CAD build for the part. Positions are in the model's coordinates, mm. Round coordinates to 2 decimals unless told otherwise and drop trailing zeros. Order: outer loops, then holes, each group sorted by start corner. A loop starts at its lowest first (then second) coordinate and runs counter-clockwise, first axis right, second up. Notation, with made-up numbers: (70.25, 65) - (88.25, 65) arc R14 ccw to (88.25, 84) - close; hole circle Ø10 at (1.25, -33.5). An arc over 180 degrees is marked (long way). Use one line per item in the form item = value. Start each with the question number.
Autodesk Inventor part; units mm, degrees
ref_plane "YZ Plane" through (0, 0, 0) normal (1, 0, 0) x (0, 1, 0)
ref_plane "XZ Plane" through (0, 0, 0) normal (0, 1, 0) x (-1, 0, 0)
ref_plane "XY Plane" through (0, 0, 0) normal (0, 0, 1) x (1, 0, 0)
sketch "Sketch1" plane through (0, 0, 0) normal (0, 0, 1) x (1, 0, 0)
  line L0 (0, 0) -> (25, 0)
  line L1 (25, 0) -> (25, 3)
  line L2 (0, 3) -> (25, 3)
  line L3 (0, 0) -> (0, 3)
  line L4 (0.2071, -72) -> (11, -72)
  line L5 (0.2071, -69) -> (11, -69)
  line L6 (25, -69) -> (50, -69)
  line L7 (25, 0) -> (50, 0)
  line L8 (-25, 0) -> (0, 0)
  line L9 (-22, 0) -> (-22, -10.8146)
  line L10 (-25, -22) -> (-25, -47)
  line L11 (-25, -47) -> (-22, -47)
  line L12 (-22, -10.8146) -> (-22, -58.1854)
  line L13 (-25, -22) -> (-22, -22)
  line L14 (-22, -58.1854) -> (-22, -69)
  line L15 (-25, -69) -> (0, -69)
  line L16 (50, 0) -> (50, -22)
  line L17 (50, -22) -> (47, -22)
  line L18 (47, -22) -> (47, -47)
  line L19 (47, -47) -> (50, -47)
  line L20 (50, -47) -> (50, -69)
  line L21 (50, 0) -> (25, 0)
  line L22 (25, 3) -> (25, 0)
  line L23 (25, 3) -> (0, 3)
  line L24 (0, 3) -> (0, 0)
  line L25 (-22, -10.8146) -> (-22, 0)
  line L26 (-22, 0) -> (0, 0)
  line L27 (-22, -22) -> (-25, -22)
  line L28 (-25, -22) -> (-25, -47)
  line L29 (-22, -47) -> (-25, -47)
  line L30 (-22, -58.1854) -> (-22, -69)
  line L31 (-22, -69) -> (0, -69)
  line L32 (0, -72) -> (0, -69)
  line L33 (0, -72) -> (25, -72)
  line L34 (25, -72) -> (25, -69)
  line L35 (25, -69) -> (50, -69)
  line L36 (11, -72) -> (11, -69)
  line L37 (0.2071, -69) -> (0.2071, -72)
  dimension "d0" = 3
extrude "Extrusion1" add sketch "Sketch1" along normal blind 3
sketch "Sketch2" plane through (0, 0, 3) normal (0, 0, 1) x (1, 0, 0)
  line L0 (-25, -22) -> (-25, -47)
  line L1 (-25, -34.5) -> (7, -34.5)
  line L2 (-25, -34.5) -> (-14, -34.5)
  circle A0 centre (-14, -34.5) radius 21
  circle A1 centre (-14, -34.5) radius 25
  point P0 (0, 0)
  dimension "d3" = 32
  dimension "d4" = 11
  dimension "d5" = 4
extrude "Extrusion2" cut sketch "Sketch2" against normal blind 20 contours A0 | A1
sketch "Sketch3" plane through (0, 0, 3) normal (0, 0, 1) x (1, 0, 0)
  line L0 (-1.2929, -65) -> (30.2929, -65)
  line L1 (-4.5, -67) -> (-4.5, -65)
  line L2 (33.5, -67) -> (33.5, -65)
  line L3 (30.6464, -65) -> (33.5, -65)
  line L4 (30.6464, -65) -> (30.2929, -65)
  line L5 (30.2929, -67) -> (30.6464, -67)
  line L6 (33.5, -67) -> (30.6464, -67)
  line L7 (30.2929, -67) -> (-1.2929, -67)
  arc A0 (-22, -58.1854) -> (-22, -10.8146) centre (-14, -34.5) ccw
  line L8 (-22, -58.1854) -> (-22, -69)
  line L9 (-22, -69) -> (0, -69)
  line L10 (0, -69) -> (0, -72)
  line L11 (50, -69) -> (50, -47)
  line L12 (50, -47) -> (47, -47)
  line L13 (47, -47) -> (47, -22)
  line L14 (47, -22) -> (50, -22)
  line L15 (50, -22) -> (50, 0)
  line L16 (50, 0) -> (25, 0)
  line L17 (25, 0) -> (25, 3)
  line L18 (25, 3) -> (0, 3)
  line L19 (0, 3) -> (0, 0)
  line L20 (0, 0) -> (-22, 0)
  line L21 (-22, 0) -> (-22, -10.8146)
  line L22 (-4.5, -65) -> (-1.6464, -65)
  line L23 (-1.2929, -65) -> (-1.6464, -65)
  line L24 (-1.6464, -67) -> (-4.5, -67)
  line L25 (-1.6464, -67) -> (-1.2929, -67)
  line L26 (0, -72) -> (25, -72)
  line L27 (25, -69) -> (50, -69)
  line L28 (25, -72) -> (25, -69)
extrude "Extrusion3" cut sketch "Sketch3" against normal blind 3 contours L0 L4 L3 L2 L6 L5 L7 L25 L24 L1 L22 L23
sketch "Sketch4" plane through (0, 0, 3) normal (0, 0, 1) x (1, 0, 0)
  line L0 (47, -47) -> (47, -22)
  line L1 (47, -34.5) -> (34.3, -34.5)
  line L2 (34.3, -34.5) -> (34.3, -36)
  line L3 (34.3, -36) -> (34.3, -33)
  line L4 (34.3, -33) -> (47, -33)
  line L5 (47, -33) -> (47, -36)
  line L6 (47, -36) -> (34.3, -36)
  line L7 (40.65, -36) -> (40.65, -38)
  line L8 (40.65, -38) -> (38.15, -38)
  line L9 (38.15, -38) -> (38.15, -31)
  line L10 (38.15, -31) -> (40.65, -31)
  line L11 (40.65, -31) -> (40.65, -36)
  line L12 (25, 3) -> (0, 3)
  line L13 (50, 0) -> (25, 0)
  line L14 (0, 0) -> (-22, 0)
  line L15 (25, -69) -> (50, -69)
  line L16 (0, -72) -> (25, -72)
  line L17 (-22, -69) -> (0, -69)
  line L18 (50, 0) -> (25, 0)
  line L19 (37.5, 0) -> (37.5, -12.7)
  line L20 (37.5, -12.7) -> (39, -12.7)
  line L21 (39, -12.7) -> (36, -12.7)
  line L22 (36, -12.7) -> (36, 0)
  line L23 (39, 0) -> (39, -12.7)
  line L24 (36, -6.35) -> (34, -6.35)
  line L25 (34, -6.35) -> (34, -8.85)
  line L26 (34, -8.85) -> (41, -8.85)
  line L27 (41, -8.85) -> (41, -6.35)
  line L28 (41, -6.35) -> (36, -6.35)
  line L29 (50, -69) -> (25, -69)
  line L30 (37.5, -69) -> (37.5, -56.3)
  line L31 (37.5, -56.3) -> (39, -56.3)
  line L32 (39, -56.3) -> (36, -56.3)
  line L33 (36, -56.3) -> (36, -69)
  line L34 (39, -69) -> (39, -56.3)
  line L35 (36, -62.65) -> (34, -62.65)
  line L36 (34, -62.65) -> (34, -60.15)
  line L37 (34, -60.15) -> (41, -60.15)
  line L38 (41, -60.15) -> (41, -62.65)
  line L39 (41, -62.65) -> (36, -62.65)
  line L40 (-4.5, -65) -> (33.5, -65)
  line L41 (33.5, -65) -> (33.5, -67)
  line L42 (33.5, -67) -> (-4.5, -67)
  line L43 (-4.5, -67) -> (-4.5, -65)
  arc A0 (-22, -58.1854) -> (-22, -10.8146) centre (-14, -34.5) ccw
  line L44 (-22, -58.1854) -> (-22, -69)
  line L45 (-22, -69) -> (0, -69)
  line L46 (0, -69) -> (0, -72)
  line L47 (0, -72) -> (25, -72)
  line L48 (25, -69) -> (50, -69)
  line L49 (50, -69) -> (50, -47)
  line L50 (50, -47) -> (47, -47)
  line L51 (47, -47) -> (47, -22)
  line L52 (47, -22) -> (50, -22)
  line L53 (50, -22) -> (50, 0)
  line L54 (50, 0) -> (25, 0)
  line L55 (25, 0) -> (25, 3)
  line L56 (25, 3) -> (0, 3)
  line L57 (0, 3) -> (0, 0)
  line L58 (0, 0) -> (-22, 0)
  line L59 (-22, 0) -> (-22, -10.8146)
  circle A1 centre (12.5, 1.5) radius 1.5
  line L60 (39, -56.3) -> (36, -56.3)
  line L61 (36, -56.3) -> (36, -69)
  line L62 (36, -69) -> (39, -69)
  line L63 (39, -69) -> (39, -56.3)
  circle A2 centre (12.5, -70.5) radius 1.5
  line L64 (25, -72) -> (25, -69)
  arc A3 (42.9741, -36.0257) -> (30.0259, -20.7829) centre (36.5, -28.4043) ccw
  line L65 (26.9692, -49.6214) -> (42.9741, -36.0257)
  arc A4 (14.0209, -34.3786) -> (26.9692, -49.6214) centre (20.4951, -42) ccw
  line L66 (30.0259, -20.7829) -> (14.0209, -34.3786)
  dimension "d10" = 12.7
  dimension "d11" = 1.5
  dimension "d12" = 3
  dimension "d13" = 2
  dimension "d14" = 2.5
  dimension "d15" = 7
  dimension "d16" = 12.7
  dimension "d17" = 1.5
  dimension "d18" = 3
  dimension "d19" = 2
  dimension "d20" = 2.5
  dimension "d21" = 7
  dimension "d22" = 3
  dimension "d25" = 3
extrude "Extrusion4" cut sketch "Sketch4" against normal blind 25.4 contours A1 | A2 | L15 L30 L39 L34 | L15 L33 L39 L30 | L39 L30 L37 L34 | L34 L37 L38 L39 | L39 L33 L37 L30 | L37 L30 L31 L34 | L35 L36 L37 L33 | L37 L33 L32 L30 | L23 L28 L19 L13 | L19 L28 L22 L13 | L28 L27 L26 L23 | L23 L26 L19 L28 | L19 L26 L22 L28 | L23 L20 L19 L26 | L22 L26 L25 L24 | L19 L21 L22 L26
sketch "Sketch5" plane through (0, 0, 3) normal (0, 0, 1) x (1, 0, 0)
  line L0 (26.9692, -49.6214) -> (42.9741, -36.0257)
  line L1 (44.9164, -38.3121) -> (28.9114, -51.9078)
  line L2 (42.9741, -36.0257) -> (44.9164, -38.3121)
  line L3 (28.9114, -51.9078) -> (26.9692, -49.6214)
  line L4 (30.0259, -20.7829) -> (14.0209, -34.3786)
  line L5 (12.0787, -32.0922) -> (28.0836, -18.4965)
  line L6 (28.0836, -18.4965) -> (30.0259, -20.7829)
  line L7 (14.0209, -34.3786) -> (12.0787, -32.0922)
  arc A0 (10.5873, -50.4164) -> (19.1404, -54.9292) centre (20.4951, -42) ccw
  line L8 (10.5873, -50.4164) -> (12.8737, -48.4741)
  arc A1 (12.8737, -48.4741) -> (19.1404, -51.9078) centre (20.4951, -42) ccw
  line L9 (19.1404, -51.9078) -> (19.1404, -54.9292)
  point P0 (0, 0)
extrude "Extrusion5" cut sketch "Sketch5" against normal blind 25.4
sketch "Sketch6" plane through (0, 3, 3) normal (0, 1, 0) x (1, 0, 0)
  line L0 (12.5, 0) -> (12.5, 3)
  line L1 (12.5, 3) -> (0, 3)
  line L2 (0, 3) -> (0, 0)
  line L3 (12.5, 0) -> (0, 0)
  line L4 (25, 0) -> (12.5, 0)
  line L5 (25, 3) -> (25, 0)
  line L6 (25, 3) -> (12.5, 3)
  point P0 (0, 3)
extrude "Extrusion6" add sketch "Sketch6" along normal blind 0.5
sketch "Sketch7" plane through (0, -72, 0) normal (0, -1, 0) x (1, 0, 0)
  line L0 (12.5, 3) -> (12.5, 0)
  line L1 (0, 3) -> (12.5, 3)
  line L2 (0, 0) -> (0, 3)
  line L3 (0, 0) -> (12.5, 0)
  line L4 (12.5, 0) -> (25, 0)
  line L5 (25, 0) -> (25, 3)
  line L6 (12.5, 3) -> (25, 3)
extrude "Extrusion7" add sketch "Sketch7" along normal blind 0.5
properties part number "pared frontal 2"
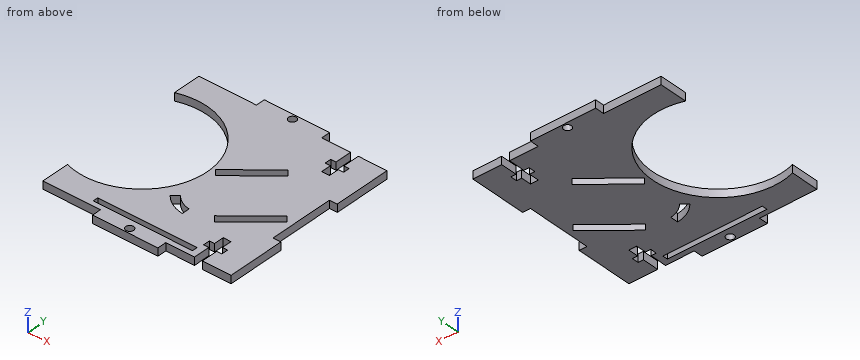
(1) Slice it at A-A (x = -14). Give the cut face in (y, z), and give its area (3 significant figures).
(2) Slice it at D-D (z = 0.75). Give the number of separate pieces and of enclosed holes in the cut face, and give its area (3 significant figures).
(3) Slice it at B-B (y = 1.5). Give the cut face in (x, z).
(4) Flat gauge pins, fed straight in: P1, Ø1.5, axis at x = 46.5, z = 2, coming from the +Y side; P2, Ø1.6, axis at x = 40.5, z = 2, coming from the -Y side; P3, Ø5, axis at x = 12.5, y = 1.5, coming from the +Z side. Where does each tip first touch, or does it go through?
(5) Slice it at C-C (x = 22.5). Give the cut face in (y, z).
(6) Wall check: line 1 (Y direction, x = 12.5, z = 2.25); line 2 (X direction, y = -66.5, z = 0.75); line 3 (Y direction, x = 13, z = 1.95). Give the ranges that are in metal, low to high. Write a range as [from, to].
Results list:
q1.outline = (-69, 0) - (-59.5, 0) - (-59.5, 3) - (-69, 3) - close; (-9.5, 0) - (0, 0) - (0, 3) - (-9.5, 3) - close
q1.area = 57.0 mm²
q2.separate_pieces = 1
q2.enclosed_holes = 6
q2.area = 3,360 mm²
q3.outline = (0, 0) - (11, 0) - (11, 3) - (0, 3) - close; (14, 0) - (25, 0) - (25, 3) - (14, 3) - close
q4.P1 = 0
q4.P2 = -69
q4.P3 = 3
q5.outline = (-72.5, 0) - (-67, 0) - (-67, 3) - (-72.5, 3) - close; (-65, 0) - (-27.18, 0) - (-27.18, 3) - (-65, 3) - close; (-23.24, 0) - (3.5, 0) - (3.5, 3) - (-23.24, 3) - close
q6.line_1 = [-72.5, -72], [-69, -67], [-65, -52.25], [-48.79, -32.59], [-31.73, 0], [3, 3.5]
q6.line_2 = [-22, -4.5], [33.5, 36], [39, 50]
q6.line_3 = [-72.5, -71.91], [-69.09, -67], [-65, -52.62], [-48.62, -33.18], [-31.31, 0.09], [2.91, 3.5]
